```python
from build123d import *

# Parameters (mm, degrees)
BOSS_EXTRUDE1_DEPTH       = 13
FILLET2_R                 = 0.5
SKETCH2_R                 = 1.6
CUT_EXTRUDE1_DEPTH        = 4.896527904
REVISION_INDICATION_DEPTH = 0.4


with BuildPart() as part:
    # Sketch1 → Boss-Extrude1 (new body)
    with BuildSketch(Plane(origin=(0, 0, 0), x_dir=(1, 0, 0), z_dir=(0, 1, 0))):
        Polygon((20.35, 0.1), (14.35, 0.1), (0, 0), (-0.016724739, 2.4), (14.35, 3.9), (20.35, 3.9), (34.716724739, 2.4), (34.7, 0), align=None)
    extrude(amount=BOSS_EXTRUDE1_DEPTH)

    # Fillet2
    fillet2_edges = [part.edges().sort_by_distance(p)[0] for p in [
        (-0.016724739, 6.5, -2.4),
        (34.716724739, 6.5, -2.4),
        (34.7, 6.5, 0),
        (0, 6.5, 0),
    ]]
    fillet(fillet2_edges, radius=FILLET2_R)

    # Sketch2 → Cut-Extrude1 (cut, through all)
    with BuildSketch(Plane(origin=(0, 0, -3.9), x_dir=(-1, 0, 0), z_dir=(0, 0, -1))):
        with Locations((-17.35, 6.5)):
            Circle(SKETCH2_R)
    extrude(amount=-CUT_EXTRUDE1_DEPTH, mode=Mode.SUBTRACT)

    # Sketch5 → revision indication (add)
    with BuildSketch(Plane(origin=(-0.248057274, 0, -2.375847049), x_dir=(-0.994593653, 0, 0.103843465), z_dir=(-0.103843465, 0, -0.994593653))):
        with BuildLine():
            add(Edge.make_bspline(
                [(-1.785308798, 1.976923077), (-1.749947985, 1.974821832), (-1.680627244, 1.970702586), (-1.580407683, 1.942442049), (-1.489703086, 1.892261337), (-1.40890887, 1.825381725), (-1.342312834, 1.744291021), (-1.290343795, 1.654309873), (-1.262329436, 1.553251269), (-1.258240196, 1.483528859), (-1.256142132, 1.44775641)],
                knots=[0, 0, 0, 0, 0.000106068, 0.000207934, 0.000309251, 0.000414952, 0.000520654, 0.000622584, 0.00072445, 0.000831784, 0.000831784, 0.000831784, 0.000831784], degree=3))
            add(Edge.make_bspline(
                [(-1.256142132, 1.44775641), (-1.258311293, 1.412843512), (-1.262588847, 1.343995789), (-1.290279579, 1.243699421), (-1.342708899, 1.153662038), (-1.408449529, 1.071471016), (-1.489723058, 1.004449722), (-1.580622123, 0.954695939), (-1.680391977, 0.924411918), (-1.749908735, 0.920554208), (-1.785308798, 0.918589744)],
                knots=[0, 0, 0, 0, 0.000104802, 0.000206668, 0.000308598, 0.000415282, 0.000520984, 0.0006223, 0.000724523, 0.000830591, 0.000830591, 0.000830591, 0.000830591], degree=3))
            add(Edge.make_bspline(
                [(-1.785308798, 0.918589744), (-1.82073437, 0.920483127), (-1.889894366, 0.924179507), (-1.989291812, 0.955317742), (-2.080744455, 1.003983162), (-2.162002161, 1.071595984), (-2.228293388, 1.153239101), (-2.278413725, 1.244319503), (-2.308512996, 1.343708683), (-2.312471536, 1.412786963), (-2.314475465, 1.44775641)],
                knots=[0, 0, 0, 0, 0.000106068, 0.000207073, 0.000309509, 0.000415211, 0.000521895, 0.000623212, 0.000725435, 0.000830237, 0.000830237, 0.000830237, 0.000830237], degree=3))
            add(Edge.make_bspline(
                [(-2.314475465, 1.44775641), (-2.312548513, 1.483587428), (-2.308786377, 1.553543092), (-2.278350536, 1.653690044), (-2.228682266, 1.744709926), (-2.161543907, 1.825258007), (-2.080764113, 1.892726399), (-1.989512426, 1.941829667), (-1.889654975, 1.970931558), (-1.820694086, 1.974891267), (-1.785308798, 1.976923077)],
                knots=[0, 0, 0, 0, 0.000107334, 0.000209557, 0.000310874, 0.000416575, 0.000522277, 0.000624713, 0.000725357, 0.000831425, 0.000831425, 0.000831425, 0.000831425], degree=3))
        make_face()
        with BuildLine():
            add(Edge.make_bspline(
                [(-4.146206234, 1.976923077), (-4.110845421, 1.974821832), (-4.04152468, 1.970702586), (-3.941305118, 1.942442049), (-3.850600522, 1.892261337), (-3.769806306, 1.825381725), (-3.70321027, 1.744291021), (-3.651241231, 1.654309873), (-3.623226872, 1.553251269), (-3.619137632, 1.483528859), (-3.617039568, 1.44775641)],
                knots=[0, 0, 0, 0, 0.000106068, 0.000207934, 0.000309251, 0.000414952, 0.000520654, 0.000622584, 0.00072445, 0.000831784, 0.000831784, 0.000831784, 0.000831784], degree=3))
            add(Edge.make_bspline(
                [(-3.617039568, 1.44775641), (-3.619208729, 1.412843512), (-3.623486283, 1.343995789), (-3.651177015, 1.243699421), (-3.703606335, 1.153662038), (-3.769346965, 1.071471016), (-3.850620494, 1.004449722), (-3.941519559, 0.954695939), (-4.041289413, 0.924411918), (-4.110806171, 0.920554208), (-4.146206234, 0.918589744)],
                knots=[0, 0, 0, 0, 0.000104802, 0.000206668, 0.000308598, 0.000415282, 0.000520984, 0.0006223, 0.000724523, 0.000830591, 0.000830591, 0.000830591, 0.000830591], degree=3))
            add(Edge.make_bspline(
                [(-4.146206234, 0.918589744), (-4.181631806, 0.920483127), (-4.250791802, 0.924179507), (-4.350189248, 0.955317742), (-4.441641891, 1.003983162), (-4.522899597, 1.071595984), (-4.589190824, 1.153239101), (-4.639311161, 1.244319503), (-4.669410431, 1.343708683), (-4.673368972, 1.412786963), (-4.675372901, 1.44775641)],
                knots=[0, 0, 0, 0, 0.000106068, 0.000207073, 0.000309509, 0.000415211, 0.000521895, 0.000623212, 0.000725435, 0.000830237, 0.000830237, 0.000830237, 0.000830237], degree=3))
            add(Edge.make_bspline(
                [(-4.675372901, 1.44775641), (-4.673445949, 1.483587428), (-4.669683813, 1.553543092), (-4.639247972, 1.653690044), (-4.589579702, 1.744709926), (-4.522441343, 1.825258007), (-4.441661549, 1.892726399), (-4.350409862, 1.941829667), (-4.25055241, 1.970931558), (-4.181591522, 1.974891267), (-4.146206234, 1.976923077)],
                knots=[0, 0, 0, 0, 0.000107334, 0.000209557, 0.000310874, 0.000416575, 0.000522277, 0.000624713, 0.000725357, 0.000831425, 0.000831425, 0.000831425, 0.000831425], degree=3))
        make_face()
        with BuildLine():
            add(Edge.make_bspline(
                [(-6.50710367, 1.976923077), (-6.471742857, 1.974821832), (-6.402422116, 1.970702586), (-6.302202554, 1.942442049), (-6.211497957, 1.892261337), (-6.130703742, 1.825381725), (-6.064107706, 1.744291021), (-6.012138667, 1.654309873), (-5.984124308, 1.553251269), (-5.980035068, 1.483528859), (-5.977937003, 1.44775641)],
                knots=[0, 0, 0, 0, 0.000106068, 0.000207934, 0.000309251, 0.000414952, 0.000520654, 0.000622584, 0.00072445, 0.000831784, 0.000831784, 0.000831784, 0.000831784], degree=3))
            add(Edge.make_bspline(
                [(-5.977937003, 1.44775641), (-5.980106165, 1.412843512), (-5.984383719, 1.343995789), (-6.012074451, 1.243699421), (-6.064503771, 1.153662038), (-6.130244401, 1.071471016), (-6.21151793, 1.004449722), (-6.302416994, 0.954695939), (-6.402186849, 0.924411918), (-6.471703607, 0.920554208), (-6.50710367, 0.918589744)],
                knots=[0, 0, 0, 0, 0.000104802, 0.000206668, 0.000308598, 0.000415282, 0.000520984, 0.0006223, 0.000724523, 0.000830591, 0.000830591, 0.000830591, 0.000830591], degree=3))
            add(Edge.make_bspline(
                [(-6.50710367, 0.918589744), (-6.542529242, 0.920483127), (-6.611689237, 0.924179507), (-6.711086684, 0.955317742), (-6.802539327, 1.003983162), (-6.883797033, 1.071595984), (-6.95008826, 1.153239101), (-7.000208597, 1.244319503), (-7.030307867, 1.343708683), (-7.034266408, 1.412786963), (-7.036270337, 1.44775641)],
                knots=[0, 0, 0, 0, 0.000106068, 0.000207073, 0.000309509, 0.000415211, 0.000521895, 0.000623212, 0.000725435, 0.000830237, 0.000830237, 0.000830237, 0.000830237], degree=3))
            add(Edge.make_bspline(
                [(-7.036270337, 1.44775641), (-7.034343385, 1.483587428), (-7.030581249, 1.553543092), (-7.000145408, 1.653690044), (-6.950477138, 1.744709926), (-6.883338779, 1.825258007), (-6.802558985, 1.892726399), (-6.711307298, 1.941829667), (-6.611449846, 1.970931558), (-6.542488958, 1.974891267), (-6.50710367, 1.976923077)],
                knots=[0, 0, 0, 0, 0.000107334, 0.000209557, 0.000310874, 0.000416575, 0.000522277, 0.000624713, 0.000725357, 0.000831425, 0.000831425, 0.000831425, 0.000831425], degree=3))
        make_face()
        with BuildLine():
            add(Edge.make_bspline(
                [(-8.868001106, 1.976923077), (-8.832640293, 1.974821832), (-8.763319552, 1.970702586), (-8.66309999, 1.942442049), (-8.572395393, 1.892261337), (-8.491601178, 1.825381725), (-8.425005142, 1.744291021), (-8.373036103, 1.654309873), (-8.345021744, 1.553251269), (-8.340932504, 1.483528859), (-8.338834439, 1.44775641)],
                knots=[0, 0, 0, 0, 0.000106068, 0.000207934, 0.000309251, 0.000414952, 0.000520654, 0.000622584, 0.00072445, 0.000831784, 0.000831784, 0.000831784, 0.000831784], degree=3))
            add(Edge.make_bspline(
                [(-8.338834439, 1.44775641), (-8.341003601, 1.412843512), (-8.345281155, 1.343995789), (-8.372971887, 1.243699421), (-8.425401207, 1.153662038), (-8.491141837, 1.071471016), (-8.572415366, 1.004449722), (-8.66331443, 0.954695939), (-8.763084284, 0.924411918), (-8.832601042, 0.920554208), (-8.868001106, 0.918589744)],
                knots=[0, 0, 0, 0, 0.000104802, 0.000206668, 0.000308598, 0.000415282, 0.000520984, 0.0006223, 0.000724523, 0.000830591, 0.000830591, 0.000830591, 0.000830591], degree=3))
            add(Edge.make_bspline(
                [(-8.868001106, 0.918589744), (-8.903426678, 0.920483127), (-8.972586673, 0.924179507), (-9.07198412, 0.955317742), (-9.163436763, 1.003983162), (-9.244694469, 1.071595984), (-9.310985696, 1.153239101), (-9.361106033, 1.244319503), (-9.391205303, 1.343708683), (-9.395163844, 1.412786963), (-9.397167773, 1.44775641)],
                knots=[0, 0, 0, 0, 0.000106068, 0.000207073, 0.000309509, 0.000415211, 0.000521895, 0.000623212, 0.000725435, 0.000830237, 0.000830237, 0.000830237, 0.000830237], degree=3))
            add(Edge.make_bspline(
                [(-9.397167773, 1.44775641), (-9.395240821, 1.483587428), (-9.391478685, 1.553543092), (-9.361042844, 1.653690044), (-9.311374574, 1.744709926), (-9.244236214, 1.825258007), (-9.16345642, 1.892726399), (-9.072204734, 1.941829667), (-8.972347282, 1.970931558), (-8.903386394, 1.974891267), (-8.868001106, 1.976923077)],
                knots=[0, 0, 0, 0, 0.000107334, 0.000209557, 0.000310874, 0.000416575, 0.000522277, 0.000624713, 0.000725357, 0.000831425, 0.000831425, 0.000831425, 0.000831425], degree=3))
        make_face()
    extrude(amount=REVISION_INDICATION_DEPTH)


solid = part.part
```
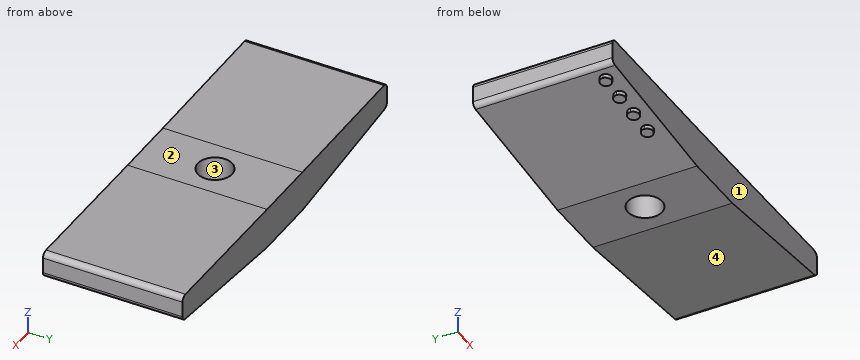
Could you check a few things on this model? Use its own coordinates, in mm. Face numbers are marked on the shaded views. Give positions to 0.01 mm unless a question says otherwise; leave off trailing zeros. Loops run counter-clockwise (first coordinate to the right, second up) from the corner with the lowest first, then second, coordinate; pieces in that order, holes last. Notation, with made-up numbers: (60, -24) -> (78, -24) arc R15 cw to (78, 3) -> close; hole circle Ø3 at (83, 3.25). An arc over 180 degrees is marked (long way). Put each result on its own line as item: value.
(1) Imagine slicing it at D-D on x = 23. Write out the boundary of the cut face in (y, z).
Computed:
outline: (0, -3.62) -> (13, -3.62) -> (13, -0.08) -> (0, -0.08) -> close
(2) Imagine slicing it at C-C on x = 27. Write out the boundary of the cut face in (y, z).
Computed:
outline: (0, -3.21) -> (13, -3.21) -> (13, -0.05) -> (0, -0.05) -> close
(3) Imagine slicing it at B-B on x = 17.35. Write out the boundary of the cut face in (y, z).
Computed:
outline: (0, -3.9) -> (4.9, -3.9) -> (4.9, -0.1) -> (0, -0.1) -> close; (8.1, -3.9) -> (13, -3.9) -> (13, -0.1) -> (8.1, -0.1) -> close
(4) I'm going to push flat-ended pins straight in: pin 1 Ø3 at (x, y) = (18.5, 8.5) entering from +Z; pin 2 Ø6 at (x, y) = (23, 10.5) entering from -Z. Where does each tip first touch, or does it pass through?
Computed:
pin 1: z = -0.1
pin 2: z = -3.9
(5) Imagine slicing it at A-A on y = 6.5. Write out the boundary of the cut face in (x, z).
Computed:
outline: (-0.01, -1.95) arc R0.5 ccw to (0.43, -2.45) -> (14.35, -3.9) -> (15.75, -3.9) -> (15.75, -0.1) -> (14.35, -0.1) -> (0.5, 0) arc R0.5 ccw to (0, -0.5) -> close; (18.95, -3.9) -> (20.35, -3.9) -> (34.27, -2.45) arc R0.5 ccw to (34.71, -1.95) -> (34.7, -0.5) arc R0.5 ccw to (34.2, 0) -> (20.35, -0.1) -> (18.95, -0.1) -> close
(6) Thinking about a two-plate mould opening in X: for the marked faces 1, 2, 3 and 4, which applies, pulls with the +X half, pulls with the -X half, needs draft (parallel to the pull), parting line crosses it, or undercut?
Computed:
face 1: needs draft
face 2: undercut
face 3: undercut
face 4: pulls with the +X half
(7) Please list where these lines run through material, in increasing order: probe 1 along Y at (x, z) = (17.35, -1); probe 2 along Z at (x, y) = (15, 2.5); probe 3 along X at (y, z) = (8.25, -1.7). Write a range as [from, to].
Computed:
probe 1: [0, 4.9], [8.1, 13]
probe 2: [-3.9, -0.1]
probe 3: [-0.01, 34.71]
